The model under review builds one solid part; all positions refer to its coordinate system, in mm. A direction names the side the tool comes from. Round coordinates to 2 decimals unless told otherwise and drop trailing zeros. Write each loop counter-clockwise with the first axis right and the second up, starting at its lowest first coordinate (ties: lowest second). Pieces come first, ordered by that corner, then holes. Notation, with made-up numbers: (8.5, 63.25) -> (44.5, 63.25) arc R11 cw to (44.5, 70.25) -> close; hole circle Ø6 at (19, 88). An arc over 180 degrees is marked (long way). Answer as a JSON object with one key per item and string values. Group by question number.
1) We need section D-D, the plane x = 13.5. Write out the cut boundary in (y, z) (3 decimals).
2) We need section A-A, the plane z = 11.75. Write out the cut boundary in (x, y).
3) Machinability: for faces 1 (the flat face through (8, -25.4, 13)), 2 (the flat face through (25.4, -19, 3)), 3 (the flat face through (16.953, -19, 9)), which of the approach directions +Z, -Z, +X, -X, +Y, -Y give a long, thin tool a straight path to every point of the face, cutting with its end or side? Answer none if there is none.
4) We need section B-B, the plane x = 6.25. Write out the cut boundary in (y, z), then the cut area to 3 significant figures.
5) Insertion check: pin 1 Ø6 at (x, y) = (8, -21.5) entering from -Z; pin 2 Ø8.5 at (x, y) = (3.5, -21.5) entering from +Z; pin 3 Ø4 at (x, z) = (6.5, 13.5) entering from -Y; pin 4 Ø7 at (y, z) = (-16.5, 11) entering from +X. Each pin has a flat end and moves straight along its axis. Give the tip position at first contact, or say it passes through.
6) To check wall thickness, follow probe 1 along Z at (x, y) = (10.5, -34.5); probe 2 along Z at (x, y) = (1, -24); probe 3 along X at (y, z) = (-14, 11.25). State the ranges of each line that lie inside material, in increasing order. Write a range as [from, to].
7) We need section C-C, the plane y = -19.5. Write out the cut boundary in (x, z) (3 decimals).
from build123d import *

# Parameters (mm, degrees)
F0_W     = 25.4
F0_H     = 6.35
F1_DEPTH = 38.1
F3_DEPTH = 12.7
F5_DEPTH = 12.7


with BuildPart() as f1:
    # F0 (on Front) → F1 (new body)
    with BuildSketch(Plane.XZ):
        with Locations((12.7, 3.175)):
            Rectangle(F0_W, F0_H)
    extrude(amount=F1_DEPTH)

    # F2 (on face) → F3 (join)
    with BuildSketch(Plane(origin=(0, 0, 0), x_dir=(-1, 0, 0), z_dir=(0, 1, 0))):
        Polygon((-25.4, 6.35), (0, 6.35), (0, 25.4), align=None)
    extrude(amount=-F3_DEPTH)

    # F4 (on face) → F5 (join)
    with BuildSketch(Plane.XZ.offset(12.7)):
        Polygon((0, 19.490924), (0, 6.35), (16.953341, 6.35), (16.953341, 12.684994), (7.878768, 19.490924), align=None)
    extrude(amount=F5_DEPTH)


solid = f1.part
Here are the results:
{
 "1": {"outline": "(-38.1, 0) -> (0, 0) -> (0, 15.275) -> (-25.4, 15.275) -> (-25.4, 6.35) -> (-38.1, 6.35) -> close"},
 "2": {"outline": "(0, -25.4) -> (16.95, -25.4) -> (16.95, -12.7) -> (18.2, -12.7) -> (18.2, 0) -> (0, 0) -> close"},
 "3": {"face 1": "+Z, +X, -X, -Y", "face 2": "+Z, -Z, +X, +Y, -Y", "face 3": "+Z, +X, -Y"},
 "4": {"outline": "(-38.1, 0) -> (0, 0) -> (0, 20.71) -> (-12.7, 20.71) -> (-12.7, 19.49) -> (-25.4, 19.49) -> (-25.4, 6.35) -> (-38.1, 6.35) -> close", "area": "591 mm^2"},
 "5": {"pin 1": "stops at z = 0", "pin 2": "stops at z = 19.49", "pin 3": "stops at y = -25.4", "pin 4": "stops at x = 16.95"},
 "6": {"probe 1": "z = [0, 6.35]", "probe 2": "z = [0, 19.49]", "probe 3": "x = [0, 16.95]"},
 "7": {"outline": "(0, 0) -> (25.4, 0) -> (25.4, 6.35) -> (16.953, 6.35) -> (16.953, 12.685) -> (7.879, 19.491) -> (0, 19.491) -> close"}
}
